Geometry: final body of the model. Coordinates: model frame, mm. A direction names the side the tool comes from. Coordinates: 2 decimals unless noted, no trailing zeros. Loops run counter-clockwise (first coordinate to the right, second up) from the corner with the lowest first, then second, coordinate; pieces in that order, holes last. Notation, with made-up numbers: (61.5, 0) - (105.5, 0) arc R38 ccw to (105.5, 39) - close; hole circle Ø2 at (29, 56.5). An arc over 180 degrees is marked (long way). Put each result on its own line as item: value. Start each with the question number.
1) Section A-A on z = 0. Output: boundary loops of the cut face in (x, y), and give its area (4 significant figures).
2) Section D-D on x = -8.25. Output: boundary loops of the cut face in (y, z), and give its area (3 significant figures).
3) Contact query for flat-ended pins moving along their axis: pin 1 Ø4 at (x, z) = (8.25, 0) entering from -Y; pin 2 Ø3 at (x, z) = (0.5, -0.5) entering from +Y; pin 3 Ø2 at (y, z) = (4, -7) entering from -X; pin 4 Ø1.5 at (x, y) = (-7.5, 1) entering from -Z. Output: stop coordinate, or through.
4) Reachability of faces 5 (the cylindrical face through (-0.325, 1.232, 9.714)), 6 (the flat face through (1.2, 2, 1.2)) from +Z, -Z, +X, -X, +Y, -Y: full face, straight path, thin tool, end or side. Return the list, or none.
5) Section B-B on x = 0. Output: boundary loops of the cut face in (y, z), and give its area (4 significant figures).
6) Material intervals for line 1 along Z through (x, y) = (0, 1.15); line 2 along X through (y, z) = (2.2, 0.25), sorted ascending. Write a range as from..to.
7) Section C-C on y = 1.4. Output: boundary loops of the cut face in (x, z).
8) Draft query along Z for faces 1 (the cylindrical face through (7.06, 1.23, 0.91)), 2 (the cylindrical face through (6.586, 1.232, -10.329)), 3 (the cylindrical face through (-0.596, 4.028, 2.685)), 4 (the flat face through (5.3, 2.5, -0.2)). Return one class per face: +Z half, -Z half, draft (parallel to the pull), parting line (faces both ways), or undercut.
```python
from build123d import *

# Parameters (mm, degrees)
SKETCH_1_R          = 12.25
EXTRUDE_1_DEPTH     = 2.5
SKETCH_1_3_R        = 5
EXTRUDE_2_DEPTH     = 6
SKETCH_2_R          = 1.5
CUT_EXTRUDE_2_DEPTH = 6
CUT_EXTRUDE_START   = 6
SKETCH_2_3_R        = 2.75
CUT_EXTRUDE_3_DEPTH = 4


with BuildPart() as part:
    # Эскиз1 → Бобышка-Вытянуть1 (new body)
    with BuildSketch(Plane(origin=(0, 0, 0), x_dir=(1, 0, 0), z_dir=(0, 1, 0))):
        Circle(SKETCH_1_R)
    extrude(amount=EXTRUDE_1_DEPTH)

    # Эскиз1<3> → Бобышка-Вытянуть2 (add)
    with BuildSketch(Plane(origin=(0, 0, 0), x_dir=(1, 0, 0), z_dir=(0, 1, 0))):
        Circle(SKETCH_1_3_R)
    extrude(amount=EXTRUDE_2_DEPTH)

    # Эскиз2 → Вырез-Вытянуть2 (cut)
    with BuildSketch(Plane(origin=(0, 0, 0), x_dir=(1, 0, 0), z_dir=(0, 1, 0))):
        Circle(SKETCH_2_R)
        with Locations((-8.25, 0)):
            Circle(SKETCH_2_R)
        with Locations((0, 8.25)):
            Circle(SKETCH_2_R)
        with Locations((8.25, 0)):
            Circle(SKETCH_2_R)
        with Locations((0, -8.25)):
            Circle(SKETCH_2_R)
    extrude(amount=CUT_EXTRUDE_2_DEPTH, mode=Mode.SUBTRACT)

    # Эскиз2<3> → Вырез-Вытянуть3 (cut)
    with BuildSketch(Plane(origin=(0, 0, 0), x_dir=(1, 0, 0), z_dir=(0, 1, 0)).offset(CUT_EXTRUDE_START)):
        Circle(SKETCH_2_3_R)
    extrude(amount=-CUT_EXTRUDE_3_DEPTH, mode=Mode.SUBTRACT)


solid = part.part
```
Answer block:
1. outline: (-12.25, 0) - (-9.75, 0) - (-9.75, 2.5) - (-12.25, 2.5) - close; (-6.75, 0) - (-1.5, 0) - (-1.5, 2) - (-2.75, 2) - (-2.75, 6) - (-5, 6) - (-5, 2.5) - (-6.75, 2.5) - close; (1.5, 0) - (6.75, 0) - (6.75, 2.5) - (5, 2.5) - (5, 6) - (2.75, 6) - (2.75, 2) - (1.5, 2) - close; (9.75, 0) - (12.25, 0) - (12.25, 2.5) - (9.75, 2.5) - close
1. area: 53.25 mm²
2. outline: (0, -9.06) - (2.5, -9.06) - (2.5, -1.5) - (0, -1.5) - close; (0, 1.5) - (2.5, 1.5) - (2.5, 9.06) - (0, 9.06) - close
2. area: 37.8 mm²
3. pin 1: stops at y = 0
3. pin 2: stops at y = 2
3. pin 3: passes through
3. pin 4: stops at z = -10.22
4. face 5: +Y, -Y
4. face 6: +Y
5. outline: (0, -12.25) - (2.5, -12.25) - (2.5, -9.75) - (0, -9.75) - close; (0, -6.75) - (2.5, -6.75) - (2.5, -5) - (6, -5) - (6, -2.75) - (2, -2.75) - (2, -1.5) - (0, -1.5) - close; (0, 1.5) - (2, 1.5) - (2, 2.75) - (6, 2.75) - (6, 5) - (2.5, 5) - (2.5, 6.75) - (0, 6.75) - close; (0, 9.75) - (2.5, 9.75) - (2.5, 12.25) - (0, 12.25) - close
5. area: 53.25 mm²
6. line 1: z = -12.25..-9.75, -6.75..-1.5, 1.5..6.75, 9.75..12.25
6. line 2: x = -12.25..-9.73, -6.77..-2.74, 2.74..6.77, 9.73..12.25
7. outline: circle Ø24.5 at (0, 0); hole circle Ø3 at (-8.25, 0); hole circle Ø3 at (0, -8.25); hole circle Ø3 at (0, 0); hole circle Ø3 at (0, 8.25); hole circle Ø3 at (8.25, 0)
8. face 1: undercut
8. face 2: parting line
8. face 3: undercut
8. face 4: draft
